Input: part model. Units: mm. Frame: model coordinates. Give positions to 0.01 mm unless a question says otherwise; leave off trailing zeros. Loops run counter-clockwise (first coordinate to the right, second up) from the corner with the lowest first, then second, coordinate; pieces in that order, holes last. Notation, with made-up numbers: (-17, 2) -> (18, 2) arc R21 cw to (18, 37) -> close; hole circle Ø5 at (69, 77.5). An arc over 180 degrees is marked (long way). Answer in a Markdown table with one row per item. Add a question column.
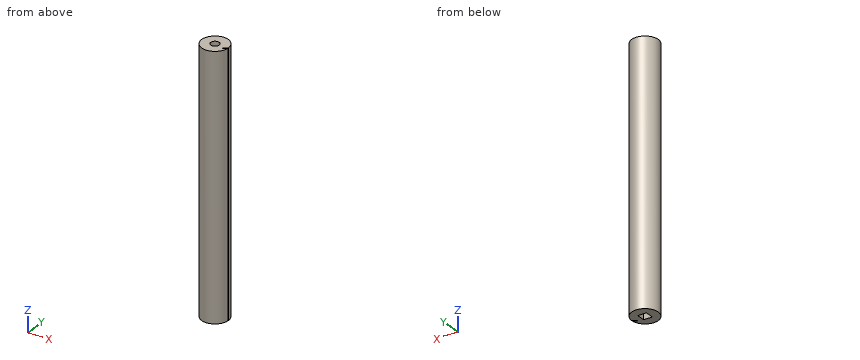
```python
from build123d import *

# Parameters (mm, degrees)
F1_DEPTH = 150
F2_R     = 2.5
F3_DEPTH = 5
F4_W     = 5
F4_H     = 5
F5_DEPTH = 5


with BuildPart() as f1:
    # F0 (on Top) → F1 (new body)
    with BuildSketch(Plane.XY):
        with BuildLine():
            Line((5.272375, -1.385031), (7.745967, 0.25))
            ThreePointArc((7.745967, 0.25), (-7.749832, 0.051027), (7.742003, -0.351977))
            Line((7.742003, -0.351977), (5.548085, -1.802145))
            Line((5.548085, -1.802145), (5.272375, -1.385031))
        make_face()
    extrude(amount=F1_DEPTH)

    # F2 (on face) → F3 (cut)
    with BuildSketch(Plane.XY.offset(150)):
        Circle(F2_R)
    extrude(amount=-F3_DEPTH, mode=Mode.SUBTRACT)

    # F4 (on face) → F5 (cut)
    with BuildSketch(Plane(origin=(0, 0, 0), x_dir=(1, 0, 0), z_dir=(0, 0, -1))):
        Rectangle(F4_W, F4_H)
    extrude(amount=-F5_DEPTH, mode=Mode.SUBTRACT)


solid = f1.part
```
1) Pin query (flat end, axial travel): pin 1 (1.5 mm diameter, centred on y = -3, z = 63, fed in from -X); pin 2 (4 mm diameter, centred on x = 3.5, z = 49, fed in from -Y); pin 3 (1.5 mm diameter, centred on x = 6, z = 107.5, fed in from +Y); pin 4 (5 mm diameter, centred on x = -1.5, z = 15.5, fed in from -Y). Return the tip coordinate at first contact, or that it passes through.
2) Material intervals for line 1 along Y through (x, z) = (0, 147.8); line 2 along X through (y, z) = (0.5, 84.5); line 3 along Y through (x, z) = (7, 127.5), sorted ascending.
3) Section A-A on x = 0. Output: boundary loops of the cut face in (y, z), and give its area (4 significant figures).
4) Section B-B on z = 41. Output: boundary loops of the cut face in (x, y), and give its area (3 significant figures).
5) Section C-C on y = 4.25. Output: boundary loops of the cut face in (x, z).
Working result:
| question | item | result |
|---|---|---|
| 1 | pin 1 | stops at x = -7.42 |
| 1 | pin 2 | stops at y = -7.6 |
| 1 | pin 3 | stops at y = 5.7 |
| 1 | pin 4 | stops at y = -7.75 |
| 2 | line 1 | y = -7.75 to -2.5, 2.5 to 7.75 |
| 2 | line 2 | x = -7.73 to 7.73 |
| 2 | line 3 | y = -3.33 to -0.84, -0.24 to 3.33 |
| 3 | outline | (-7.75, 0) -> (-2.5, 0) -> (-2.5, 5) -> (2.5, 5) -> (2.5, 0) -> (7.75, 0) -> (7.75, 150) -> (2.5, 150) -> (2.5, 145) -> (-2.5, 145) -> (-2.5, 150) -> (-7.75, 150) -> close |
| 3 | area | 2,275 mm2 |
| 4 | outline | (5.27, -1.39) -> (7.75, 0.25) arc R7.75 ccw (long way) to (7.74, -0.35) -> (5.55, -1.8) -> close |
| 4 | area | 187 mm2 |
| 5 | outline | (-6.48, 0) -> (6.48, 0) -> (6.48, 150) -> (-6.48, 150) -> close |
